Can you work these out from the drawing? Everything is in mm from the part's minimum corner. Round coordinates to 2 decimals unless told otherwise and drop trailing zeros. Loops run counter-clockwise (first coordinate to the right, second up) from the corner with the lowest first, then second, coordinate; pieces in that order, holes last. Notation, with made-up numbers: M 72,27 L 128,27 A19 ccw 128,56 Z; hole C -9,19 d9. An arc over 180 degrees is marked long. Answer in a Markdown table with one row per item.
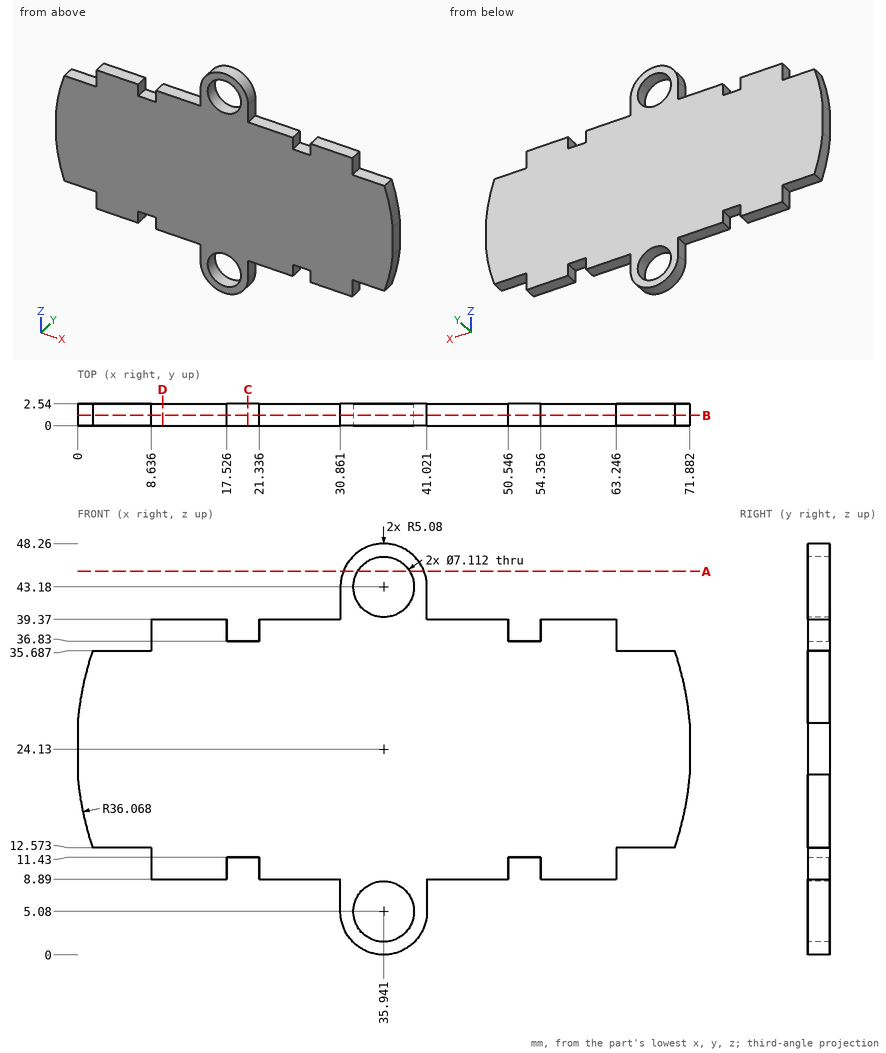
1) I want a section at D-D, the plane x = 10. Please give me the cut outline in (y, z), plus the area to 3 significant figures.
Computed:
| item | result |
|---|---|
| outline | M 0,8.89 L 2.54,8.89 L 2.54,39.37 L 0,39.37 Z |
| area | 77.4 mm² |
2) I want a section at B-B, the plane y = 1.2. State how many separate pieces and enclosed holes the cut face has, plus the area to 3 significant figures.
Computed:
| item | result |
|---|---|
| separate pieces | 1 |
| enclosed holes | 2 |
| area | 2,080 mm² |
3) Will these pins go through, and if not, where does the flat tip stop? P1, Ø1.3, axis at x = 5, y = 1.5, coming from the +Z side; P2, Ø0.8, axis at y = 1, z = 10, coming from the +X side; P3, Ø1.3, axis at x = 19, y = 2, coming from the +Z side.
Computed:
| item | result |
|---|---|
| P1 | stops at z = 35.69 |
| P2 | stops at x = 63.25 |
| P3 | stops at z = 36.83 |
4) I want a section at C-C, the plane x = 20. Please give me the cut outline in (y, z).
Computed:
| item | result |
|---|---|
| outline | M 0,11.43 L 2.54,11.43 L 2.54,36.83 L 0,36.83 Z |
5) I want a section at A-A, the plane z = 45. Please give me the cut outline in (x, y), plus the area to 3 significant figures.
Computed:
| item | result |
|---|---|
| outline | M 31.2,0 L 32.89,0 L 32.89,2.54 L 31.2,2.54 Z; M 39,0 L 40.68,0 L 40.68,2.54 L 39,2.54 Z |
| area | 8.57 mm² |
6) I need wall thicknesses on line 1 (X direction, y = 0.8, z = 9.5); line 2 (X direction, y = 2.3, z = 43.5); line 3 (Z direction, x = 33, y = 1.3). Which ranges of each line are inside material? Lowest first, please.
Computed:
| item | result |
|---|---|
| line 1 | x = 8.64 to 17.53, 21.34 to 50.55, 54.36 to 63.25 |
| line 2 | x = 30.87 to 32.4, 39.48 to 41.01 |
| line 3 | z = 0.94 to 3.08, 7.08 to 41.18, 45.18 to 47.32 |
